```python
from build123d import *

# Parameters (mm, degrees)
EXTRUDE_THIN1_DEPTH      = 100
SKETCH2_W                = 50
SKETCH2_H                = 30
REVOLVE1_ANGLE           = 180
SKETCH3_R                = 27.5
CUT_EXTRUDE1_DEPTH       = 351.89172119
CUT_EXTRUDE1_DEPTH_BACK  = 351.89172119
SKETCH4_R                = 70
BOSS_EXTRUDE1_DEPTH      = 65
BOSS_EXTRUDE1_DEPTH_BACK = 30
SKETCH5_R                = 50
CUT_EXTRUDE2_DEPTH       = 364.765034054
SKETCH6_R                = 15
CUT_EXTRUDE3_DEPTH       = 347.446244026
RIB1_REACH               = 348.699
SKETCH8_WALL_W           = 749.740096374
SKETCH8_WALL_H           = 20
RIB23_REACH              = 348.699
SKETCH15_WALL_W          = 778.361425474
SKETCH15_WALL_H          = 20


with BuildPart() as part:
    # Sketch1 → Extrude-Thin1 (new body)
    with BuildSketch(Plane.XY):
        Polygon((-15, 80), (-15, -15), (280, -15), (280, 15), (15, 15), (15, 80), align=None)
    extrude(amount=EXTRUDE_THIN1_DEPTH)

    # Sketch2 → Revolve1 (revolve)
    with BuildSketch(Plane(origin=(280, 0, 0), x_dir=(0, 0, -1), z_dir=(1, 0, 0))):
        with Locations((-75, 0)):
            Rectangle(SKETCH2_W, SKETCH2_H)
    revolve(axis=Axis((280, 15, 50), (0, 1, 0)), revolution_arc=REVOLVE1_ANGLE)

    # Sketch3 → Cut-Extrude1 (cut, two sides)
    with BuildSketch(Plane(origin=(0, 15, 0), x_dir=(1, 0, 0), z_dir=(0, 1, 0))) as cut_extrude1_sk:
        with Locations(Location((280, -50, 0), (0, 0, 270))):
            Circle(SKETCH3_R)
    extrude(amount=CUT_EXTRUDE1_DEPTH, mode=Mode.SUBTRACT)
    extrude(cut_extrude1_sk.sketch, amount=-CUT_EXTRUDE1_DEPTH_BACK, mode=Mode.SUBTRACT)

    # Sketch4 → Boss-Extrude1 (add, two sides)
    with BuildSketch(Plane(origin=(0, 15, 0), x_dir=(1, 0, 0), z_dir=(0, 1, 0))) as boss_extrude1_sk:
        with Locations(Location((139.34266344, -50, 0), (0, 0, 270))):
            Circle(SKETCH4_R)
    extrude(amount=BOSS_EXTRUDE1_DEPTH)
    extrude(boss_extrude1_sk.sketch, amount=-BOSS_EXTRUDE1_DEPTH_BACK)

    # Sketch5 → Cut-Extrude2 (cut, through all)
    with BuildSketch(Plane(origin=(0, 80, 0), x_dir=(1, 0, 0), z_dir=(0, 1, 0))):
        with Locations(Location((139.34266344, -50, 0), (0, 0, 270))):
            Circle(SKETCH5_R)
    extrude(amount=-CUT_EXTRUDE2_DEPTH, mode=Mode.SUBTRACT)

    # Sketch6 → Cut-Extrude3 (cut, through all)
    with BuildSketch(Plane(origin=(15, 0, 0), x_dir=(0, 0, -1), z_dir=(1, 0, 0))):
        with Locations((-79.487733911, 47.5)):
            Circle(SKETCH6_R)
        with Locations(Location((-20.512266089, 47.5, 0), (0, 0, 180))):
            Circle(SKETCH6_R)
    extrude(amount=-CUT_EXTRUDE3_DEPTH, mode=Mode.SUBTRACT)

    # Sketch8 wall → Rib1 (add, up to next)
    with BuildSketch(Plane(origin=(42.17133172, 80, 50), x_dir=(1, 0, 0), z_dir=(0, 1, 0)), mode=Mode.PRIVATE) as rib1_sk1:
        Rectangle(SKETCH8_WALL_W, SKETCH8_WALL_H)
    rib1_tool1 = extrude(rib1_sk1.sketch, amount=-RIB1_REACH, mode=Mode.PRIVATE) - part.part
    add(rib1_tool1.solids().sort_by_distance((42.17133172, 80, 50))[0])

    # Sketch15 wall → Rib23 (add, up to next)
    with BuildSketch(Plane(origin=(223.056644771, 43.396320835, 50), x_dir=(0.470501542113, -0.88239917207, 0), z_dir=(0.88239917207, 0.470501542113, 0)), mode=Mode.PRIVATE) as rib23_sk1:
        Rectangle(SKETCH15_WALL_W, SKETCH15_WALL_H)
    rib23_tool1 = extrude(rib23_sk1.sketch, amount=-RIB23_REACH, mode=Mode.PRIVATE) - part.part
    add(rib23_tool1.solids().sort_by_distance((223.056644771, 43.396320835, 50))[0])


solid = part.part
```
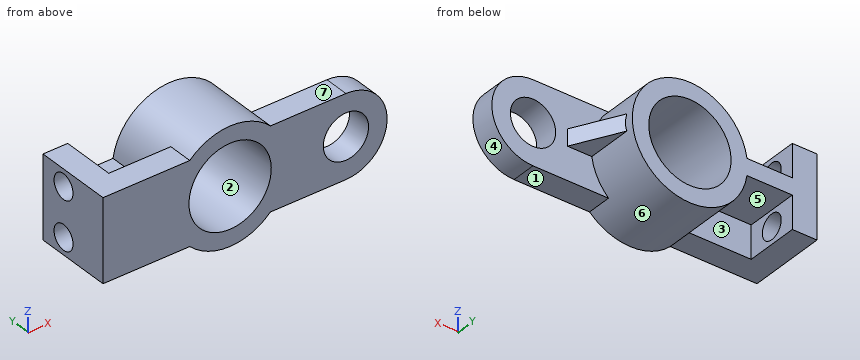
Source: CAD feature listing. Evaluate the final solid. Frame: model axes, mm. Face numbers are marked on the shaded views. A direction names the side the tool comes from. Round coordinates to 2 decimals unless told otherwise and drop trailing zeros. Loops run counter-clockwise (first coordinate to the right, second up) from the corner with the lowest first, then second, coordinate; pieces in that order, holes last.
1. Section query C-C on z = 68.5. Output: boundary loops of the cut face in (x, y).
2. Section query B-B on x = 268.5. Output: boundary loops of the cut face in (y, z), and give its area (3 significant figures).
3. Contact query for flat-ended pins moving along their axis: pin 1 (20 mm diameter, centred on y = 57, z = 71.5, fed in from +X); pin 2 (9 mm diameter, centred on x = 217.5, y = 46.5, fed in from -Z); pin 3 (8 mm diameter, centred on x = 130.5, z = 92, fed in from +Y); pin 4 (15 mm diameter, centred on x = 221, y = 49.5, fed in from +Z). Output: stop coordinate, or through.
4. Section query D-D on y = 20. Output: boundary loops of the cut face in (x, z).
5. Ray query, L1, parallel to X at y = 10, z = 50; L2, parallel to Z at x = 5, y = 47; L3, parallel to X at y = 62, z = 87. Return the intervals inside material, ascending.
6. Section query A-A on y = 47.5. Output: boundary loops of the cut face in (x, z), and give its area (3 significant figures).
7. Mould query, pull axis X, two halves, no side actions, for the marked faces 1, 2, 3 and 4. Classes: released by +X, released by -X, zero draft, split by the parting line, or undercut.
8. Access query for the marked faces 5, 6 and 7. Directions: +Z, -Z, +X, -X, +Y, -Y. A direction counts if a zero-diameter tool reaches every point of the face in a straight line with its end or side. Return the directions, or none.
Answers below:
1. outline: (-15, -15) - (92.89, -15) - (92.89, 80) - (71.83, 80) - (71.83, 15) - (15, 15) - (15, 37.29) - (-15, 37.29) - close; (-15, 57.71) - (15, 57.71) - (15, 80) - (-15, 80) - close; (185.79, -15) - (259.65, -15) - (259.65, 15) - (206.85, 15) - (206.85, 80) - (185.79, 80) - close; (300.35, -15) - (326.45, -15) - (326.45, 15) - (300.35, 15) - close
2. outline: (-15, 0) - (15, 0) - (15, 25.02) - (-15, 25.02) - close; (-15, 74.98) - (15, 74.98) - (15, 100) - (-15, 100) - close
2. area: 1,500 mm2
3. pin 1: stops at x = 208.39
3. pin 2: stops at z = 40
3. pin 3: passes through
3. pin 4: stops at z = 60
4. outline: (-15, 0) - (15, 0) - (15, 40) - (70.06, 40) arc R70 ccw to (208.62, 40) - (235.53, 40) - (235.53, 60) - (208.62, 60) arc R70 ccw to (70.06, 60) - (15, 60) - (15, 100) - (-15, 100) - close; hole circle Ø100 at (139.34, 50)
5. L1: x = -15 to 89.34, 189.34 to 252.5, 307.5 to 330
5. L2: z = 0 to 5.52, 35.5 to 64.5, 94.48 to 100
5. L3: x = -15 to 15, 79.92 to 105.71, 172.97 to 198.76
6. outline: (-15, 0) - (15, 0) - (15, 5.51) - (-15, 5.51) - close; (-15, 35.51) - (15, 35.51) - (15, 40) - (70.06, 40) arc R70 ccw to (208.62, 40) - (220.87, 40) - (220.87, 60) - (208.62, 60) arc R70 ccw to (70.06, 60) - (15, 60) - (15, 64.49) - (-15, 64.49) - close; (-15, 94.49) - (15, 94.49) - (15, 100) - (-15, 100) - close; hole circle Ø100 at (139.34, 50)
6. area: 10,100 mm2
7. face 1: zero draft
7. face 2: undercut
7. face 3: undercut
7. face 4: released by +X
8. face 5: -Z, +Y
8. face 6: +Y
8. face 7: +Z, +X, +Y, -Y
